Check sheet for the modelled part. Datum: model origin and axes. Units: mm. A direction names the side the tool comes from. Round coordinates to 2 decimals unless told otherwise and drop trailing zeros. Write each loop counter-clockwise with the first axis right and the second up, starting at its lowest first coordinate (ties: lowest second). Pieces come first, ordered by that corner, then holes.
Item 1: Material ranges on line 1 along Y through (x, z) = (9, 132.08); line 2 along Z through (x, y) = (9.75, -26.5); line 3 along Z through (x, y) = (4.5, -17.5), recorded low to high.
Item 2: Release check for a two-part mould opening along Y. For faces 4 (the flat face through (6.26, -10.23, 63.34)), 5 (the flat face through (6, 44.45, 76)), 6 (the flat face through (12.7, -9, -37)) record: pulls with the +Y half, pulls with the -Y half, needs draft (parallel to the pull), parting line crosses it, or undercut.
Item 3: Section check A-A, the plane z = 59.5. Record the cut outline in (x, y).
Item 4: Depth check by flat-ended pin: pin 1 (6.5 mm diameter, centred on x = 7.5, y = -2, fed in from -Z); pin 2 (4 mm diameter, centred on x = 11, y = 30, fed in from +Z); pin 3 (4 mm diameter, centred on x = 5, y = -1, fed in from +Z). Enter the tip coordinate at first touch or a pass-through.
Item 5: Section check C-C, the plane z = 132.08. Record the cut outline in (x, y).
Item 6: Section check B-B, the plane x = 10.5. State how many separate pieces and enclosed holes the cut face has, plus the area to 3 significant figures.
Item 7: Set-up check for faces 1 (the cylindrical face through (6.26, -27.59, -87.16)), 2 (the flat face through (6, 38.1, -13)), 3 (the flat face through (6, -38.1, -160)): record each of +Z, -Z, +X, -X, +Y, -Y from which the full face is reachable in a straight line by a thin tool's end or side.
from build123d import *

# Parameters (mm, degrees)
SKETCH1_W               = 355.6
SKETCH1_H               = 76.2
BOSS_EXTRUDE1_DEPTH     = 12.7
CUT_EXTRUDE1_DEPTH      = 183.279291199
CUT_EXTRUDE1_DEPTH_BACK = 183.279291199
SKETCH3_W               = 76.2
SKETCH3_H               = 6.35
BOSS_EXTRUDE2_DEPTH     = 12.7
SKETCH4_W               = 12.7
SKETCH4_H               = 25.4
CUT_EXTRUDE2_DEPTH      = 184.711546997
SKETCH5_R               = 6.99999997
CUT_EXTRUDE3_DEPTH      = 184.711546997
CUT_EXTRUDE4_DEPTH      = 184.711546997
BOSS_EXTRUDE3_DEPTH     = 12.7
SKETCH9_R               = 1.27
CUT_EXTRUDE6_DEPTH      = 184.711546997
CUT_EXTRUDE7_DEPTH      = 184.711546997
FILLET1_R               = 2.54
FILLET2_R               = 2.54
SKETCH11_R              = 6.99999997
CUT_EXTRUDE8_DEPTH      = 184.711546997


with BuildPart() as part:
    # Sketch1 → Boss-Extrude1 (new body)
    with BuildSketch(Plane(origin=(0, 0, 0), x_dir=(0, 0, -1), z_dir=(1, 0, 0))):
        Rectangle(SKETCH1_W, SKETCH1_H)
    extrude(amount=BOSS_EXTRUDE1_DEPTH)

    # Sketch2 → Cut-Extrude1 (cut, two sides: drawn at the far end of the back side and taken through both)
    with BuildSketch(Plane(origin=(12.7, 0, 0), x_dir=(0, 0, -1), z_dir=(1, 0, 0)).offset(-CUT_EXTRUDE1_DEPTH_BACK)):
        Polygon((-507.550847217, -697.601694433), (-177.8, -38.1), (-139.7, 38.1), (190.050847217, 697.601694433), (-1128.95254165, 1357.103388866), (-1826.554236083, -38.1), align=None)
    extrude(amount=CUT_EXTRUDE1_DEPTH + CUT_EXTRUDE1_DEPTH_BACK, mode=Mode.SUBTRACT)

    # Sketch3 → Boss-Extrude2 (add)
    with BuildSketch(Plane.ZY):
        with Locations((-102.87, -41.275)):
            Rectangle(SKETCH3_W, SKETCH3_H)
        with Locations((76.2, -41.275)):
            Rectangle(SKETCH3_W, SKETCH3_H)
        with Locations((-102.87, 41.275)):
            Rectangle(SKETCH3_W, SKETCH3_H)
        with Locations((76.2, 41.275)):
            Rectangle(SKETCH3_W, SKETCH3_H)
    extrude(amount=-BOSS_EXTRUDE2_DEPTH)

    # Sketch4 → Cut-Extrude2 (cut, through all)
    with BuildSketch(Plane.ZY):
        with Locations((-171.45, 0)):
            Rectangle(SKETCH4_W, SKETCH4_H)
    extrude(amount=-CUT_EXTRUDE2_DEPTH, mode=Mode.SUBTRACT)

    # Sketch5 → Cut-Extrude3 (cut, through all)
    with BuildSketch(Plane.ZY):
        with Locations((-102.87, 0)):
            Circle(SKETCH5_R)
    extrude(amount=-CUT_EXTRUDE3_DEPTH, mode=Mode.SUBTRACT)

    # Sketch6 → Cut-Extrude4 (cut, through all)
    with BuildSketch(Plane.ZY):
        Polygon((-13.335, -7.08207294), (-50.428802297, -25.4), (23.758802297, -25.4), align=None)
        Polygon((-27.676197703, 0), (-64.77, 18.31792706), (-64.77, -18.31792706), align=None)
        Polygon((23.758802297, 25.4), (-50.428802297, 25.4), (-13.335, 7.08207294), align=None)
        Polygon((38.1, -18.31792706), (38.1, 18.31792706), (1.006197703, 0), align=None)
        Polygon((105.319743879, -31.75), (82.55, -8.980256121), (59.780256121, -31.75), align=None)
        Polygon((114.3, 22.769743879), (91.530256121, 0), (114.3, -22.769743879), align=None)
        Polygon((73.569743879, 0), (50.8, 22.769743879), (50.8, -22.769743879), align=None)
        Polygon((105.319743879, 31.75), (59.780256121, 31.75), (82.55, 8.980256121), align=None)
    extrude(amount=-CUT_EXTRUDE4_DEPTH, mode=Mode.SUBTRACT)

    # Sketch8 → Boss-Extrude3 (add)
    with BuildSketch(Plane(origin=(12.7, 0, 0), x_dir=(0, 0, -1), z_dir=(1, 0, 0))):
        Polygon((-147.390774674, 22.718450651), (-170.109225326, -22.718450651), (-175.788837989, -19.87864432), (-153.070387337, 25.558256983), align=None)
    extrude(amount=-BOSS_EXTRUDE3_DEPTH)

    # Sketch9 → Cut-Extrude6 (cut, through all)
    with BuildSketch(Plane.ZY):
        with Locations((-165.998025612, 11.801974388)):
            Circle(SKETCH9_R)
        with Locations((-165.998025612, -11.801974388)):
            Circle(SKETCH9_R)
        with Locations((-141.868025612, 38.998025612)):
            Circle(SKETCH9_R)
        with Locations((-141.868025612, -38.998025612)):
            Circle(SKETCH9_R)
        with Locations((-63.871974388, -38.998025612)):
            Circle(SKETCH9_R)
        with Locations((-63.871974388, 38.998025612)):
            Circle(SKETCH9_R)
        with Locations((37.201974388, 38.998025612)):
            Circle(SKETCH9_R)
        with Locations((37.201974388, -38.998025612)):
            Circle(SKETCH9_R)
        with Locations((115.198025612, -38.998025612)):
            Circle(SKETCH9_R)
        with Locations((115.198025612, 38.998025612)):
            Circle(SKETCH9_R)
        with Locations((147.792383937, 23.92327844)):
            Circle(SKETCH9_R)
        with Locations((171.314053114, -23.120059914)):
            Circle(SKETCH9_R)
    extrude(amount=-CUT_EXTRUDE6_DEPTH, mode=Mode.SUBTRACT)

    # Sketch10 → Cut-Extrude7 (cut, through all)
    with BuildSketch(Plane.ZY):
        with BuildLine():
            Line((-130.36630657, -15.875), (-114.431439115, -6.674999985))
            ThreePointArc((-114.431439115, -6.674999985), (-116.21999997, 0), (-114.431439115, 6.674999985))
            Line((-114.431439115, 6.674999985), (-130.36630657, 15.875))
            ThreePointArc((-130.36630657, 15.875), (-134.62, 0), (-130.36630657, -15.875))
        make_face()
        with BuildLine():
            ThreePointArc((-91.308560885, -6.674999985), (-96.195000015, -11.561439115), (-102.87, -13.34999997))
            Line((-102.87, -13.34999997), (-102.87, -31.75))
            ThreePointArc((-102.87, -31.75), (-86.995, -27.49630657), (-75.37369343, -15.875))
            Line((-75.37369343, -15.875), (-91.308560885, -6.674999985))
        make_face()
        with BuildLine():
            Line((-102.87, 31.75), (-102.87, 13.34999997))
            ThreePointArc((-102.87, 13.34999997), (-96.195000015, 11.561439115), (-91.308560885, 6.674999985))
            Line((-91.308560885, 6.674999985), (-75.37369343, 15.875))
            ThreePointArc((-75.37369343, 15.875), (-86.995, 27.49630657), (-102.87, 31.75))
        make_face()
        Polygon((158.000484171, -12.7), (120.65, 31.75), (120.65, -12.7), align=None)
    extrude(amount=-CUT_EXTRUDE7_DEPTH, mode=Mode.SUBTRACT)

    # Fillet1
    fillet1_edges = [part.edges().sort_by_distance(p)[0] for p in [
        (6.35, 15.875, -130.36630657),
        (6.35, -15.875, -130.36630657),
        (6.35, -31.75, -102.87),
        (6.35, -15.875, -75.37369343),
        (6.35, 15.875, -75.37369343),
        (6.35, 31.75, -102.87),
    ]]
    fillet(fillet1_edges, radius=FILLET1_R)

    # Fillet2
    fillet2_edges = [part.edges().sort_by_distance(p)[0] for p in [
        (6.35, -31.75, 105.319743879),
        (6.35, -31.75, 59.780256121),
        (6.35, -8.980256121, 82.55),
        (6.35, 0, 1.006197703),
        (6.35, 18.31792706, 38.1),
        (6.35, -18.31792706, 38.1),
        (6.35, 0, -27.676197703),
        (6.35, -18.31792706, -64.77),
        (6.35, 18.31792706, -64.77),
        (6.35, 25.4, -50.428802297),
        (6.35, 25.4, 23.758802297),
        (6.35, 7.08207294, -13.335),
        (6.35, 31.75, 59.780256121),
        (6.35, 31.75, 105.319743879),
        (6.35, 0, 73.569743879),
        (6.35, -22.769743879, 50.8),
        (6.35, 22.769743879, 50.8),
        (6.35, -22.769743879, 114.3),
        (6.35, 0, 91.530256121),
        (6.35, 22.769743879, 114.3),
        (6.35, -25.4, 23.758802297),
        (6.35, -25.4, -50.428802297),
        (6.35, -7.08207294, -13.335),
        (6.35, -12.7, 158.000484171),
        (6.35, -12.7, 120.65),
        (6.35, 31.75, 120.65),
    ]]
    fillet(fillet2_edges, radius=FILLET2_R)

    # Sketch11 → Cut-Extrude8 (cut, through all)
    with BuildSketch(Plane(origin=(12.7, 0, 0), x_dir=(0, 0, -1), z_dir=(1, 0, 0))):
        with Locations((-132.08, -25.4)):
            Circle(SKETCH11_R)
    extrude(amount=-CUT_EXTRUDE8_DEPTH, mode=Mode.SUBTRACT)


solid = part.part
Values found:
1. line 1: y = -38.1 to -32.4, -18.4 to -12.7, 18.15 to 38.1
1. line 2: z = -177.8 to -102.87, -85.38 to 65.03, 100.07 to 125.17, 138.99 to 172
1. line 3: z = -177.8 to -102.87, -76.51 to -34.43, 7.76 to 50.95, 56.07 to 74.03, 91.07 to 109.03, 114.15 to 174.6
2. face 4: undercut
2. face 5: pulls with the +Y half
2. face 6: needs draft
3. outline: (0, -44.45) - (12.7, -44.45) - (12.7, -14.07) - (0, -14.07) - close; (0, 14.07) - (12.7, 14.07) - (12.7, 44.45) - (0, 44.45) - close
4. pin 1: stops at z = -165.1
4. pin 2: stops at z = 144.75
4. pin 3: stops at z = 167.35
5. outline: (0, -38.1) - (12.7, -38.1) - (12.7, -32.4) - (0, -32.4) - close; (0, -18.4) - (12.7, -18.4) - (12.7, -12.7) - (0, -12.7) - close; (0, 18.15) - (12.7, 18.15) - (12.7, 38.1) - (0, 38.1) - close
6. separate pieces: 1
6. enclosed holes: 14
6. area: 20,500 mm2
7. face 1: +X, -X
7. face 2: +X, -X, +Y
7. face 3: -Z, +X, -X, -Y
